Can you work these out from the model? Positions are in its coordinate system, mm. Face numbers are marked on the shaded views. A direction names the side the tool comes from. Round coordinates to 2 decimals unless told otherwise and drop trailing zeros. Write each loop counter-clockwise with the first axis right and the second up, starting at its lowest first coordinate (ties: lowest second). Pieces come first, ordered by that corner, then holes. Notation, with made-up numbers: (60, 86) -> (105, 86) arc R25 ccw to (105, 125) -> close; hole circle Ø11 at (-24.75, 73). An arc over 180 degrees is marked (long way). Write item = value, one per line. Start each with the question number.
1) If I drill on line 1 (Z direction, x = 12.7, y = -13.75); line 2 (Y direction, x = 39.5, z = 3.5); line 3 (Z direction, x = 69.5, y = -2.5), over which ranges is the centre line in solid material (lowest first)?
2) Imagine slicing it at D-D, the plane x = 51. Please give me the cut outline in (y, z).
3) Imagine slicing it at B-B, the plane y = -8.75. Please give me the cut outline in (x, z), then the cut area to 3 significant figures.
4) Imagine slicing it at C-C, the plane z = 31.5. Please give me the cut outline in (x, y).
5) For the marked faces 1, 2 and 3, which set-ups out of +Z, -Z, +X, -X, +Y, -Y let a thin tool reach every point of the face, with its end or its side?
6) I'm going to push flat-ended pins straight in: pin 1 (6 mm diameter, centred on x = 40.5, y = -12, fed in from -Z); pin 2 (5 mm diameter, centred on x = 17, y = -8.5, fed in from +Z); pin 3 (6 mm diameter, centred on y = -9.5, z = 21, fed in from +X); pin 4 (2 mm diameter, centred on x = 66.5, y = -22, fed in from +Z). Where does each tip first touch, or does it pass through?
7) Imagine slicing it at A-A, the plane z = 9. Please give me the cut outline in (x, y), then the cut area to 3 significant figures.
8) Thinking about a two-plate mould opening in X: for the marked faces 4, 5 and 6, which applies, +X half, -X half, draft (parallel to the pull), parting line (faces both ways), or undercut?
from build123d import *

# Parameters (mm, degrees)
F0_W      = 76.2
F0_H      = 38.1
F1_DEPTH  = 25.4
F2_W      = 50.8
F2_H      = 24.5972746
F3_DEPTH  = 25.4
F4_R      = 6.35
F5_DEPTH  = 25.4
F7_DEPTH  = 25.4
F9_DEPTH  = 25.4
F11_DEPTH = 25.4


with BuildPart() as f1:
    # F0 (on Front) → F1 (new body)
    with BuildSketch(Plane.XZ):
        with Locations((38.1, 19.05)):
            Rectangle(F0_W, F0_H)
    extrude(amount=F1_DEPTH)

    # F2 (on face) → F3 (cut)
    with BuildSketch(Plane.XZ.offset(25.4)):
        with Locations((50.8, 25.8013627)):
            Rectangle(F2_W, F2_H)
    extrude(amount=-F3_DEPTH, mode=Mode.SUBTRACT)

    # F4 (on face) → F5 (cut)
    with BuildSketch(Plane.XZ.offset(25.4)):
        with Locations((12.7, 28.6956075579)):
            Circle(F4_R)
    extrude(amount=-F5_DEPTH, mode=Mode.SUBTRACT)

    # F6 (on face) → F7 (cut)
    with BuildSketch(Plane.XZ.offset(25.4)):
        with BuildLine():
            ThreePointArc((0, 25.4), (3.7197438789, 34.3802561211), (12.7, 38.1))
            Line((12.7, 38.1), (0, 38.1))
            Line((0, 38.1), (0, 25.4))
        make_face()
        with BuildLine():
            ThreePointArc((12.7, 38.1), (21.6802561211, 34.3802561211), (25.4, 25.4))
            Line((25.4, 25.4), (25.4, 38.1))
            Line((25.4, 38.1), (12.7, 38.1))
        make_face()
    extrude(amount=-F7_DEPTH, mode=Mode.SUBTRACT)

    # F8 (on face) → F9 (cut)
    with BuildSketch(Plane.XY.offset(13.5027254)):
        with BuildLine():
            ThreePointArc((63.5, 0), (72.4802561211, -3.7197438789), (76.2, -12.7))
            Line((76.2, -12.7), (76.2, 0))
            Line((76.2, 0), (63.5, 0))
        make_face()
        with BuildLine():
            ThreePointArc((76.2, -12.7), (72.4802561211, -21.6802561211), (63.5, -25.4))
            Line((63.5, -25.4), (76.2, -25.4))
            Line((76.2, -25.4), (76.2, -12.7))
        make_face()
    extrude(amount=-F9_DEPTH, mode=Mode.SUBTRACT)

    # F10 (on face) → F11 (cut)
    with BuildSketch(Plane.XY.offset(13.5027254)):
        with BuildLine():
            ThreePointArc((63.480662017, -19.0383808314), (67.9750906946, -17.1887647294), (69.8384103307, -12.7))
            ThreePointArc((69.8384103307, -12.7), (68.2043841634, -8.4521517018), (64.1448012955, -6.3944725193))
            Line((64.1448012955, -6.3944725193), (62.8336159646, -6.3967169))
            ThreePointArc((62.8336159646, -6.3967169), (57.1698759562, -13.0239986283), (63.480662017, -19.0383808314))
        make_face()
        with BuildLine():
            Line((38.1, -18.9609461011), (63.480662017, -19.0383808314))
            ThreePointArc((63.480662017, -19.0383808314), (57.1698759562, -13.0239986283), (62.8336159646, -6.3967169))
            Line((62.8336159646, -6.3967169), (38.1, -6.4390538989))
            ThreePointArc((38.1, -6.4390538989), (42.534090263, -8.269048665), (44.3716722533, -12.7))
            ThreePointArc((44.3716722533, -12.7), (42.534090263, -17.130951335), (38.1, -18.9609461011))
        make_face()
        with BuildLine():
            ThreePointArc((38.1, -6.4390538989), (31.8497617067, -12.7), (38.1, -18.9609461011))
            ThreePointArc((38.1, -18.9609461011), (42.534090263, -17.130951335), (44.3716722533, -12.7))
            ThreePointArc((44.3716722533, -12.7), (42.534090263, -8.269048665), (38.1, -6.4390538989))
        make_face()
    extrude(amount=-F11_DEPTH, mode=Mode.SUBTRACT)


solid = f1.part
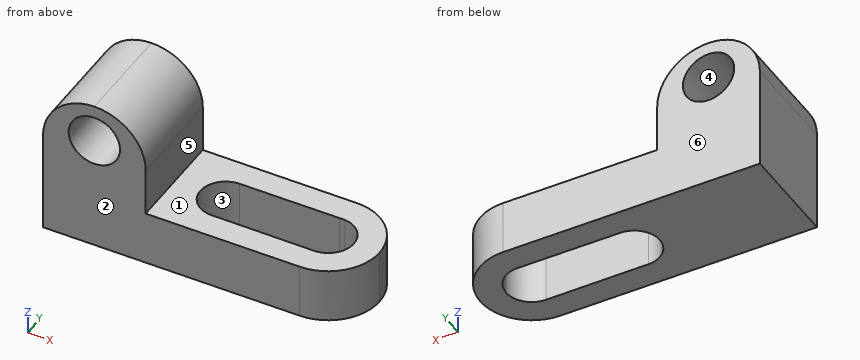
Reported:
q1.line_1 = 0 to 22.35, 35.05 to 38.1
q1.line_2 = -25.4 to -18.97, -6.44 to 0
q1.line_3 = 0 to 13.5
q2.outline = (-25.4, 0) -> (-19, 0) -> (-19, 13.5) -> (-25.4, 13.5) -> close; (-6.42, 0) -> (0, 0) -> (0, 13.5) -> (-6.42, 13.5) -> close
q3.outline = (0, 0) -> (33.25, 0) -> (33.25, 13.5) -> (25.4, 13.5) -> (25.4, 25.4) arc R12.7 ccw to (0, 25.4) -> close; (68.46, 0) -> (75.57, 0) -> (75.57, 13.5) -> (68.46, 13.5) -> close; hole circle Ø12.7 at (12.7, 28.7)
q3.area = 974 mm²
q4.outline = (1.56, -25.4) -> (7, -25.4) -> (7, 0) -> (1.56, 0) -> close; (18.4, -25.4) -> (23.84, -25.4) -> (23.84, 0) -> (18.4, 0) -> close
q5.face_1 = +Z, +X, +Y, -Y
q5.face_2 = +Z, -Z, +X, -X, -Y
q5.face_3 = +Z, -Z
q6.pin_1 = through
q6.pin_2 = 37.97
q6.pin_3 = 25.4
q6.pin_4 = 13.5
q7.outline = (0, -25.4) -> (63.5, -25.4) arc R12.7 ccw to (63.5, 0) -> (0, 0) -> close; hole (38.1, -18.96) -> (63.48, -19.04) arc R6.34 ccw to (64.14, -6.39) -> (38.1, -6.44) arc R6.26 ccw to start
q7.area = 1,420 mm²
q8.face_4 = undercut
q8.face_5 = +X half
q8.face_6 = draft
